from build123d import *

# Parameters (mm, degrees)
F0_W     = 698.5
F0_H     = 635
F1_DEPTH = 10.16
F3_R     = 5.07999
F5_D     = 15.24


# Not quite as in the source:
# - a fillet or chamfer is up to 0.001 mm smaller than in the source, because OpenCascade refuses the exact size


with BuildPart() as f1:
    # F0 (on Front) → F1 (new body)
    with BuildSketch(Plane.XZ):
        with Locations((349.25, 317.5)):
            Rectangle(F0_W, F0_H)
    extrude(amount=F1_DEPTH)

    # F3 (radius 5.08 in the source; OpenCascade refuses exactly that, so slightly less here)
    f3_edges = [f1.edges().sort_by_distance(p)[0] for p in [
        (349.25, -10.16, 635),
        (349.25, 0, 635),
        (349.25, -10.16, 0),
        (349.25, 0, 0),
    ]]
    fillet(f3_edges, radius=F3_R)

    # F5 (through all)
    with Locations(Plane.XZ.offset(10.16)):
        with Locations((431.8, 528.32), (266.7, 528.32), (596.9, 528.32), (596.9, 106.68), (431.8, 106.68), (266.7, 106.68)):
            Hole(F5_D / 2)


solid = f1.part
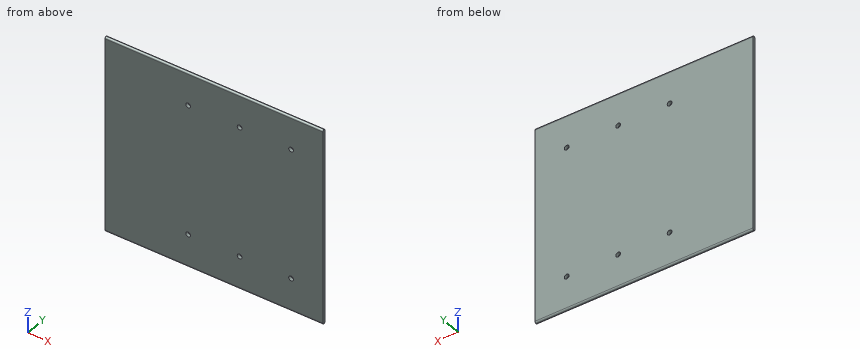
Source: CAD feature listing. Evaluate the final solid. Frame: model axes, mm. Coordinates: 2 decimals unless noted, no trailing zeros. Loops run counter-clockwise (first coordinate to the right, second up) from the corner with the lowest first, then second, coordinate; pieces in that order, holes last. Notation, with made-up numbers: (-3, 86) - (50, 86) arc R36 ccw to (50, 123) - close; hole circle Ø3 at (-36.5, 26). An arc over 180 degrees is marked (long way). One line per item, written item: value. Start each with the question number.
1. Section B-B (x = 266.7). State how many separate pieces and enclosed holes the cut face has, and give its area (3 significant figures).
2. Ray query, L1, parallel to X at y = -6, z = 528.32; L2, parallel to Z at x = 266.7, y = -5.5; L3, parallel to Z at x = 596.9, y = -3.75. Return the intervals inside material, ascending.
3. Contact query for a flat-ended pin moving along its axis: P1, Ø12, axis at x = 266.7, z = 106.68, coming from the +Y side. Output: stop coordinate, or through.
4. Section A-A (z = 106.68). Return the cut outline in (x, y), and give its area (3 significant figures).
Verdict:
1. separate pieces: 3
1. enclosed holes: 0
1. area: 6,120 mm2
2. L1: x = 0 to 259.08, 274.32 to 424.18, 439.42 to 589.28, 604.52 to 698.5
2. L2: z = 0.02 to 99.06, 114.3 to 520.7, 535.94 to 634.98
2. L3: z = 0.18 to 99.06, 114.3 to 520.7, 535.94 to 634.82
3. P1: passes through
4. outline: (0, -10.16) - (259.08, -10.16) - (259.08, 0) - (0, 0) - close; (274.32, -10.16) - (424.18, -10.16) - (424.18, 0) - (274.32, 0) - close; (439.42, -10.16) - (589.28, -10.16) - (589.28, 0) - (439.42, 0) - close; (604.52, -10.16) - (698.5, -10.16) - (698.5, 0) - (604.52, 0) - close
4. area: 6,630 mm2
